```python
from build123d import *

# Parameters (mm, degrees)
SKETCH_1_R          = 2
EXTRUDE_1_DEPTH     = 36
CUT_EXTRUDE_1_DEPTH = 6


with BuildPart() as part:
    # 草图1 → 凸台-拉伸1 (new body)
    with BuildSketch(Plane.XY):
        Circle(SKETCH_1_R)
    extrude(amount=-EXTRUDE_1_DEPTH)

    # 草图2 → 旋转1 (revolve)
    with BuildSketch(Plane(origin=(0, 0, 0), x_dir=(0, 0, -1), z_dir=(1, 0, 0))):
        with BuildLine():
            Line((35, 0), (40, 0))
            ThreePointArc((40, 0), (39.121320344, -2.121320344), (37, -3))
            Line((37, -3), (35, -3))
            Line((35, -3), (35, 0))
        make_face()
    revolve(axis=Axis((0, 0, -35), (0, 0, -1)))

    # 草图3 → 旋转2 (revolve)
    with BuildSketch(Plane(origin=(0, 0, 0), x_dir=(0, 0, -1), z_dir=(1, 0, 0))):
        Polygon((0, 2), (0, 0), (2, 0), (2, 2.1), align=None)
    revolve(axis=Axis((0, 0, -2), (0, 0, 1)))

    # 草图4 → 切除-拉伸1 (cut)
    with BuildSketch(Plane.XY):
        with BuildLine():
            Line((-0.4, -2.061552813), (-0.4, 2.061552813))
            ThreePointArc((-0.4, 2.061552813), (0, 2.1), (0.4, 2.061552813))
            Line((0.4, 2.061552813), (0.4, -2.061552813))
            ThreePointArc((0.4, -2.061552813), (0, -2.1), (-0.4, -2.061552813))
        make_face()
    extrude(amount=-CUT_EXTRUDE_1_DEPTH, mode=Mode.SUBTRACT)


solid = part.part
```
Check sheet for the modelled part. Datum: model origin and axes. Units: mm. A direction names the side the tool comes from. Give positions to 0.01 mm unless a question says otherwise; leave off trailing zeros. Write each loop counter-clockwise with the first axis right and the second up, starting at its lowest first coordinate (ties: lowest second). Pieces come first, ordered by that corner, then holes.
Item 1: Cross-section at B-B (y = 0). Enter the section's corners in (x, z), and give its area (3 significant figures).
Item 2: Cross-section at A-A (x = 0). Enter the section's corners in (y, z).
Item 3: Scan lines: L1, parallel to Z at x = -1, y = 0.5; L2, parallel to Z at x = 0, y = 0; L3, parallel to X at y = 0.75, z = -31. Record each from-to range of solid material in increasing order.
Item 4: Access from +Z, -Z, +X, -X, +Y, -Y to the whole of each face (thin tool, end or side, straight path). Record for faces 5 (the face through (1, 0, 0)), 6 (the face through (0, -2, -18)), 7 (the face through (-0.4, 0, -3)).
Item 5: Cross-section at C-C (z = -2.5). Enter the section's corners in (x, y).
Item 6: Draft check along X on faces 1 (the face through (0.4, 0, -3)), 2 (the face through (2, -1, -35)), 3 (the face through (0, 0, -6)), 4 (the face through (0, 3, -36)). Enter one of: released by +X, released by -X, zero draft, split by the parting line, or undercut.
Item 7: Gauge pin test, flat ends, axial feed: pin 1 (2 mm diameter, centred on x = -1.5, y = 2, fed in from -Z); pin 2 (1 mm diameter, centred on y = 2, z = -14, fed in from -X); pin 3 (3.5 mm diameter, centred on y = 1, z = -3.5, fed in from +X). Record the tip position at first contact, or that the pin passes through.
Item 8: Cross-section at D-D (z = -8.5). Enter the section's corners in (x, y), and give its area (3 significant figures).
Report:
1. outline: (-3, -37) arc R3 ccw to (3, -37) - (3, -35) - (2, -35) - (2, -2) - (2.1, -2) - (2, 0) - (0.4, 0) - (0.4, -6) - (-0.4, -6) - (-0.4, 0) - (-2, 0) - (-2.1, -2) - (-2, -2) - (-2, -35) - (-3, -35) - close
1. area: 162 mm2
2. outline: (-3, -37) arc R3 ccw to (3, -37) - (3, -35) - (2, -35) - (2, -6) - (-2, -6) - (-2, -35) - (-3, -35) - close
3. L1: z = -39.78 to 0
3. L2: z = -40 to -6
3. L3: x = -1.85 to 1.85
4. face 5: +Z, +X, -X, +Y, -Y
4. face 6: none
4. face 7: +Z, +Y, -Y
5. outline: (-0.4, -1.96) - (-0.4, 1.96) arc R2 ccw to start; (0.4, -1.96) arc R2 ccw to (0.4, 1.96) - close
6. face 1: undercut
6. face 2: zero draft
6. face 3: undercut
6. face 4: split by the parting line
7. pin 1: stops at z = -39.6
7. pin 2: stops at x = -1.32
7. pin 3: stops at x = 2.1
8. outline: circle Ø4 at (0, 0)
8. area: 12.6 mm2
